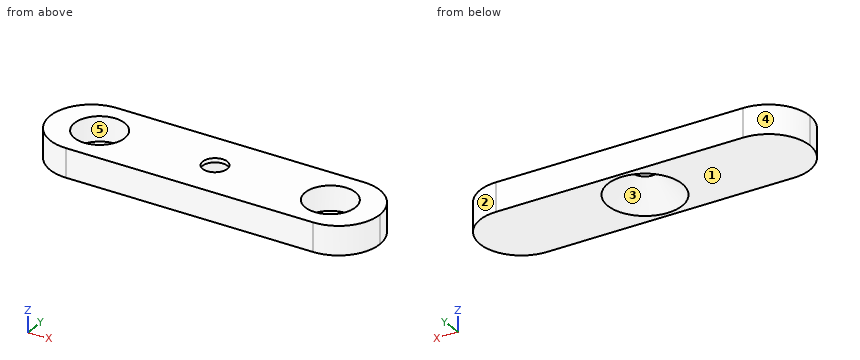
from build123d import *

# Parameters (mm, degrees)
F0_W     = 40
F0_H     = 10
F0_R     = 3.05
F0_R_2   = 1.5
F1_DEPTH = 0.5
F2_DEPTH = 3.5
F3_R     = 4.99999
F4_SIZE  = 3


# Not quite as in the source:
# - a fillet or chamfer is up to 0.001 mm smaller than in the source, because OpenCascade refuses the exact size


with BuildPart() as f1:
    # F0 (on Top) → F1 (new body)
    with BuildSketch(Plane.XY):
        Rectangle(F0_W, F0_H)
        with Locations((-14, 0)):
            Circle(F0_R, mode=Mode.SUBTRACT)
        Circle(F0_R_2, mode=Mode.SUBTRACT)
        with Locations((14, 0)):
            Circle(F0_R, mode=Mode.SUBTRACT)
        with Locations((-14, 0)):
            Circle(F0_R)
        with Locations((14, 0)):
            Circle(F0_R)
    extrude(amount=F1_DEPTH)

    # F0 (on Top) → F2 (join)
    with BuildSketch(Plane.XY):
        Rectangle(F0_W, F0_H)
        with Locations((-14, 0)):
            Circle(F0_R, mode=Mode.SUBTRACT)
        Circle(F0_R_2, mode=Mode.SUBTRACT)
        with Locations((14, 0)):
            Circle(F0_R, mode=Mode.SUBTRACT)
    extrude(amount=F2_DEPTH)

    # F3 (radius 5 in the source; OpenCascade refuses exactly that, so slightly less here)
    f3_edges = [f1.edges().sort_by_distance(p)[0] for p in [
        (20, 5, 1.75),
        (20, -5, 1.75),
        (-20, -5, 1.75),
        (-20, 5, 1.75),
    ]]
    fillet(f3_edges, radius=F3_R)

    # F4
    f4_edges = [f1.edges().sort_by_distance(p)[0] for p in [
        (-1.5, 0, 0),
    ]]
    chamfer(f4_edges, length=F4_SIZE)


solid = f1.part
Can you work these out from the model? Positions are in its coordinate system, mm. Face numbers are marked on the shaded views. A direction names the side the tool comes from. Coordinates: 2 decimals unless noted, no trailing zeros. Order: outer loops, then holes, each group sorted by start corner. A loop starts at its lowest first (then second) coordinate and runs counter-clockwise, first axis right, second up. Notation, with made-up numbers: (75.5, -5) - (82.5, -5) arc R31 cw to (82.5, 32) - close; hole circle Ø5 at (-4.75, 78.5). An arc over 180 degrees is marked (long way). Answer as a JSON object with one key per item and string values. Group by question number.
Q1. Will these pins go through, and if not, where does the flat tip stop? P1, Ø5, axis at x = -14, y = 0, coming from the +Z side; P2, Ø1, axis at y = 4, z = 2, coming from the +X side; P3, Ø3, axis at x = 3, y = 2, coming from the -Z side.
Q2. On a 3-axis mill with a long thin cutter (end or side, diameter ignored), from which of +Z, -Z, +X, -X, +Y, -Y can I reach the whole of each face in a straight line? I mean the marked faces 4 and 5. Say none if no direction works.
Q3. I need wall thicknesses on line 1 (X direction, y = 0, z = 2.9); line 2 (X direction, y = -1.5, z = 1.1); line 3 (Y direction, x = 0, z = 3.2). Which ranges of each line are inside material? Lowest first, please. Write a range as from..to.
Q4. Imagine slicing it at A-A (z = 2.2). Give the number of separate pieces and of enclosed holes in the cut face, and give its area (3 significant figures).
Q5. We'd pull the mould along X, two halves only. Please class the marked faces 1, 2 and 3: +X half, -X half, draft (parallel to the pull), parting line (faces both ways), or undercut.
Q6. Imagine slicing it at D-D (x = -12). Please give me the cut outline in (y, z).
Q7. Imagine slicing it at C-C (x = 14). Please give me the cut outline in (y, z).
Q8. Imagine slicing it at B-B (x = 0). Please give me the cut outline in (y, z).
Determined:
{
 "1": {"P1": "stops at z = 0.5", "P2": "stops at x = 18.57", "P3": "stops at z = 0"},
 "2": {"face 4": "+Z, -Z, -X, +Y", "face 5": "+Z"},
 "3": {"line 1": "x = -20..-17.05, -10.95..-1.6, 1.6..10.95, 17.05..20", "line 2": "x = -19.77..-16.66, -11.34..-3.05, 3.05..11.34, 16.66..19.77", "line 3": "y = -5..-1.5, 1.5..5"},
 "4": {"separate pieces": "1", "enclosed holes": "3", "area": "303 mm2"},
 "5": {"face 1": "draft", "face 2": "+X half", "face 3": "undercut"},
 "6": {"outline": "(-5, 0) - (5, 0) - (5, 3.5) - (2.3, 3.5) - (2.3, 0.5) - (-2.3, 0.5) - (-2.3, 3.5) - (-5, 3.5) - close"},
 "7": {"outline": "(-5, 0) - (5, 0) - (5, 3.5) - (3.05, 3.5) - (3.05, 0.5) - (-3.05, 0.5) - (-3.05, 3.5) - (-5, 3.5) - close"},
 "8": {"outline": "(-5, 0) - (-4.5, 0) - (-1.5, 3) - (-1.5, 3.5) - (-5, 3.5) - close; (1.5, 3) - (4.5, 0) - (5, 0) - (5, 3.5) - (1.5, 3.5) - close"}
}
